Answer from the drawing. Dimensions are ordinates in mm from the lowest x, y and z of the part. A direction names the side the tool comes from. Coordinates: 2 decimals unless noted, no trailing zeros. Loops run counter-clockwise (first coordinate to the right, second up) from the corner with the lowest first, then second, coordinate; pieces in that order, holes last. Notation, with made-up numbers: M 39.5,25.25 L 67.5,25.25 A27 cw 67.5,61.25 Z; hole C 27.25,-37.75 d11. An arc over 180 degrees is marked long. Put each result on its own line as item: value.
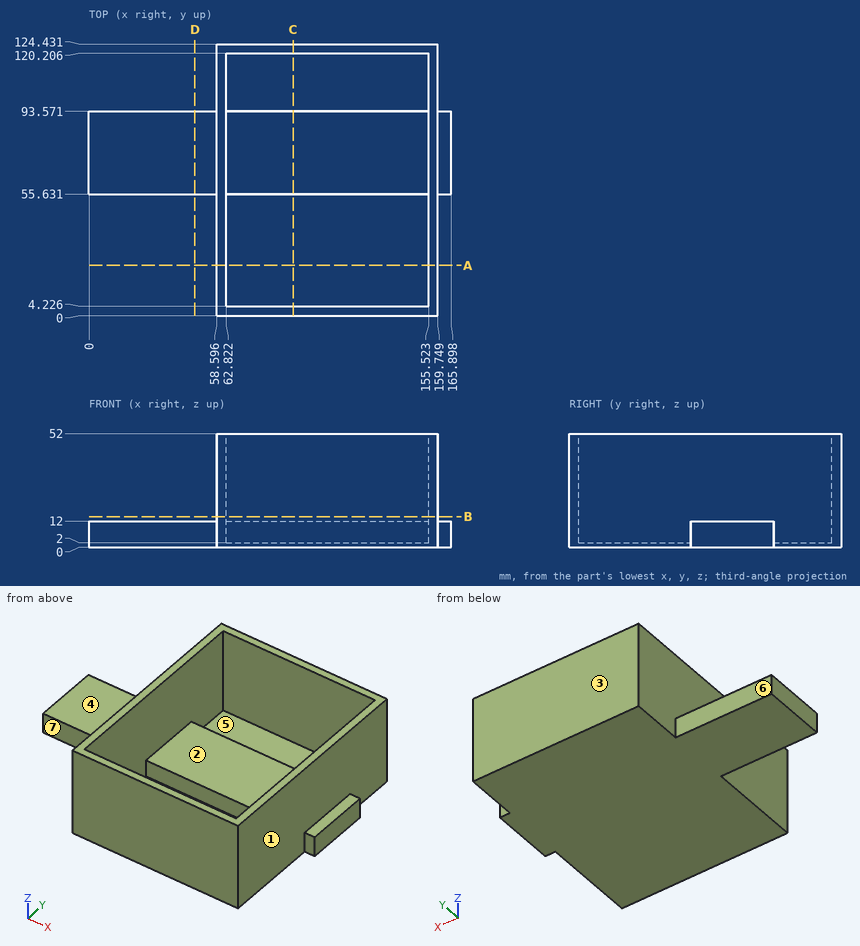
1) Find section B-B, the plane z = 14. Write down the section's boundary in (x, y) (1 decimal).
Answer list:
outline: M 58.6,0 L 159.7,0 L 159.7,124.4 L 58.6,124.4 Z; hole M 62.8,4.2 L 155.5,4.2 L 155.5,120.2 L 62.8,120.2 Z
2) Find section A-A, the plane y = 23. Write down the section's boundary in (x, z).
Answer list:
outline: M 58.6,0 L 159.75,0 L 159.75,52 L 155.52,52 L 155.52,2 L 62.82,2 L 62.82,52 L 58.6,52 Z
3) Find section C-C, the plane x = 93.5. Write down the section's boundary in (y, z) (1 decimal), plus the area to 3 significant figures.
Answer list:
outline: M 0,0 L 124.4,0 L 124.4,52 L 120.2,52 L 120.2,2 L 93.6,2 L 93.6,12 L 55.6,12 L 55.6,2 L 4.2,2 L 4.2,52 L 0,52 Z
area: 1,050 mm^2
4) Which of the six approach directions +Z, -Z, +X, -X, +Y, -Y give full straight-line access (tool end or side, diameter ignored) to the marked faces 4, 5, 6 and 7?
Answer list:
face 4: +Z, -X, +Y, -Y
face 5: +Z
face 6: +Z, -Z, -X, +Y
face 7: +Z, -Z, -X, -Y
5) Given pin 1 Ø11.5 at (x, y) = (109, 68) entering from +Z; pin 2 Ø7 at (x, z) = (164, 7.5) entering from -Y; pin 3 Ø9.5 at (x, z) = (23, 4) entering from +Y, each flat-ended and moving along its own axis, determine where each tip first touches the part or whether it passes through.
Answer list:
pin 1: stops at z = 12
pin 2: stops at y = 55.63
pin 3: stops at y = 93.57
6) Straight lines are drawn through the part: line 1 (Y direction, x = 137, z = 2.5) (1 decimal); line 2 (X direction, y = 44.5, z = 46.5); line 3 (Y direction, x = 90, z = 23) (1 decimal). For each, find the intervals that lie inside material, in ascending order. Write a range as [from, to].
Answer list:
line 1: y = [0, 4.2], [55.6, 93.6], [120.2, 124.4]
line 2: x = [58.6, 62.82], [155.52, 159.75]
line 3: y = [0, 4.2], [120.2, 124.4]
7) Determine the mould class of the marked faces 1, 2 and 3 for opening direction Y: released by +Y, released by -Y, zero draft, split by the parting line, or undercut.
Answer list:
face 1: zero draft
face 2: undercut
face 3: released by +Y
8) Find section D-D, the plane x = 48.5. Write down the section's boundary in (y, z).
Answer list:
outline: M 55.63,0 L 93.57,0 L 93.57,12 L 55.63,12 Z
